Geometry check sheet. Reference: the model listing, model coordinates, mm. A direction names the side the tool comes from. Give positions to 0.01 mm unless a question says otherwise; leave off trailing zeros. Order: outer loops, then holes, each group sorted by start corner. A loop starts at its lowest first (then second) coordinate and runs counter-clockwise, first axis right, second up.
```python
from build123d import *

# Parameters (mm, degrees)
SCHIZZO1_W                   = 60
SCHIZZO1_H                   = 60
ESTRUSIONE_ESTRUSIONE1_DEPTH = 10


with BuildPart() as part:
    # Schizzo1 → Estrusione-Estrusione1 (new body)
    with BuildSketch(Plane.XY):
        Rectangle(SCHIZZO1_W, SCHIZZO1_H)
        Polygon((7.725424859, -23.776412907), (25, 0), (7.725424859, 23.776412907), (-20.225424859, 14.694631307), (-20.225424859, -14.694631307), align=None, mode=Mode.SUBTRACT)
    extrude(amount=ESTRUSIONE_ESTRUSIONE1_DEPTH)


solid = part.part
```
Q1. Access from +Z, -Z, +X, -X, +Y, -Y to the whole of each face (thin tool, end or side, straight path). Record for faces 1 (the face through (30, 0, 5)), 2 (the face through (-20.225, 0, 5)).
Q2. Cross-section at B-B, the plane x = 5. Record the boundary of the cut face in (y, z), and give its area (3 significant figures).
Q3. Gauge pin test, flat ends, axial feed: P1, Ø4, axis at x = -22.5, y = 24, coming from the -Z side; P2, Ø2, axis at x = -8, y = 16, coming from the -Z side. Record the tip position at first contact, or that the pin passes through.
Q4. Cross-section at C-C, the plane z = 5.25. Record the boundary of the cut face in (x, y).
Q5. Thickness scan on L1, parallel to Y at x = 9, z = 5; L2, parallel to Y at x = -19, z = 4.5; L3, parallel to X at y = 5.5, z = 6.75. Record the ranges inside material, lowest first.
Q6. Cross-section at A-A, the plane y = -7.5. Record the boundary of the cut face in (x, z).
Q7. Release check for a two-part mould opening along X. For faces 3 (the face through (-30, 0, 5)), 4 (the face through (-6.45, -19.17, 4.93)), 5 (the face through (16.242, -12.055, 4.93)), 6 (the face through (0, 30, 5)) record: pulls with the +X half, pulls with the -X half, needs draft (parallel to the pull), parting line crosses it, or undercut.
Answers follow:
1. face 1: +Z, -Z, +X, +Y, -Y
1. face 2: +Z, -Z
2. outline: (-30, 0) - (-22.89, 0) - (-22.89, 10) - (-30, 10) - close; (22.89, 0) - (30, 0) - (30, 10) - (22.89, 10) - close
2. area: 142 mm2
3. P1: stops at z = 0
3. P2: passes through
4. outline: (-30, -30) - (30, -30) - (30, 30) - (-30, 30) - close; hole (-20.23, -14.69) - (7.73, -23.78) - (25, 0) - (7.73, 23.78) - (-20.23, 14.69) - close
5. L1: y = -30 to -22.02, 22.02 to 30
5. L2: y = -30 to -15.09, 15.09 to 30
5. L3: x = -30 to -20.23, 21 to 30
6. outline: (-30, 0) - (-20.23, 0) - (-20.23, 10) - (-30, 10) - close; (19.55, 0) - (30, 0) - (30, 10) - (19.55, 10) - close
7. face 3: pulls with the -X half
7. face 4: undercut
7. face 5: undercut
7. face 6: needs draft
